Here's how the part is built. I have some questions about the finished solid (model axes, mm). A direction names the side the tool comes from. Round coordinates to 2 decimals unless told otherwise and drop trailing zeros. Order: outer loops, then holes, each group sorted by start corner. A loop starts at its lowest first (then second) coordinate and runs counter-clockwise, first axis right, second up. Notation, with made-up numbers: (20, 14.25) -> (34, 14.25) arc R9 cw to (34, 29.25) -> close; hole circle Ø2 at (-37.5, 38.25). An arc over 180 degrees is marked (long way). Use a Markdown table: item, result. Add a question column.
(1) I want a section at B-B, the plane y = 26. Please give me the cut outline in (x, z), then the cut area to 3 significant figures.
(2) On a 3-axis mill with a long thin cutter (end or side, diameter ignored), from which of +Z, -Z, +X, -X, +Y, -Y can I reach the whole of each face in a straight line? I mean faces 1 (the face through (0, 0, 0)), 2 (the face through (0, 24.1, 0)), 3 (the face through (-2.22, 29.96, 1.15)), 4 (the face through (-2.44, 13.22, -0.54)). Say none if no direction works.
(3) I want a section at D-D, the plane y = 32.1. Please give me the cut outline in (x, z), then the cut area to 3 significant figures.
(4) Thinking about a two-plate mould opening in Y: for faces 5 (the face through (-0.703, 1.663, 1.696)), 6 (the face through (0, 23.997, 3)), 7 (the face through (-1.664, 32.4, -0.954)), which applies, pulls with the +Y half, pulls with the -Y half, needs draft (parallel to the pull), parting line crosses it, or undercut?
(5) I'm going to push flat-ended pins straight in: P1, Ø1.5, axis at x = -1, y = 11, coming from the -Z side; P2, Ø3, axis at y = 12, z = 1, coming from the -X side; P3, Ø2, axis at y = 25.5, z = -3, coming from the +X side. Where does each tip first touch, or does it pass through?
(6) I want a section at C-C, the plane x = 0. Please give me the cut outline in (y, z), then the cut area to 3 significant figures.
(7) I want a section at A-A, the plane z = 0. Please give me the cut outline in (x, y).
(8) If I drill on probe 1 along Y at (x, z) = (-1.2, 0); probe 2 along X at (y, z) = (29, -0.25); probe 3 along Z at (x, y) = (2.15, 32.1), over which ranges is the centre line in solid material (lowest first)?
from build123d import *

# Parameters (mm, degrees)
SKETCH1_R           = 2.5
BOSS_EXTRUDE1_DEPTH = 36.1
SKETCH2_W           = 1.7
SKETCH2_H           = 6.818294784
CUT_EXTRUDE1_DEPTH  = 12
SKETCH3_R           = 1
CUT_EXTRUDE2_DEPTH  = 6
CHAMFER1_SIZE       = 1.1
CHAMFER1_SIZE2      = 4.2
SKETCH5_W           = 4
SKETCH5_H           = 1.5


with BuildPart() as part:
    # Sketch1 → Boss-Extrude1 (new body)
    with BuildSketch(Plane(origin=(0, 0, 0), x_dir=(1, 0, 0), z_dir=(0, 1, 0))):
        with Locations(Location((0, 0, 0), (0, 0, 270))):
            Circle(SKETCH1_R)
    extrude(amount=BOSS_EXTRUDE1_DEPTH)

    # Sketch2 → Cut-Extrude1 (cut)
    with BuildSketch(Plane(origin=(0, 36.1, 0), x_dir=(1, 0, 0), z_dir=(0, 1, 0))):
        Rectangle(SKETCH2_W, SKETCH2_H)
    extrude(amount=-CUT_EXTRUDE1_DEPTH, mode=Mode.SUBTRACT)

    # Sketch3 → Cut-Extrude2 (cut, symmetric)
    with BuildSketch(Plane(origin=(-0.85, 0, 0), x_dir=(0, 0, -1), z_dir=(1, 0, 0))):
        with Locations((0, 32.1)):
            Circle(SKETCH3_R)
    extrude(amount=CUT_EXTRUDE2_DEPTH, both=True, mode=Mode.SUBTRACT)

    # Chamfer1
    chamfer1_edges = [part.edges().sort_by_distance(p)[0] for p in [
        (0, 0, -2.5),
    ]]
    chamfer1_side = [part.faces().sort_by_distance(p)[0] for p in [
        (0, 0, 0),
    ]]
    chamfer(chamfer1_edges, length=CHAMFER1_SIZE, length2=CHAMFER1_SIZE2, reference=chamfer1_side[0])

    # Sketch5 → Revolve1 (revolve)
    with BuildSketch(Plane(origin=(0, 0, 0), x_dir=(0, 0, -1), z_dir=(1, 0, 0))):
        with Locations((-4.5, 23.247432375)):
            Rectangle(SKETCH5_W, SKETCH5_H)
    revolve(axis=Axis((0, 50, 0), (0, -1, 0)))


solid = part.part
Taken from the geometry:
| question | item | result |
|---|---|---|
| 1 | outline | (-0.85, -2.35) -> (-0.85, 2.35) arc R2.5 ccw to start; (0.85, -2.35) arc R2.5 ccw to (0.85, 2.35) -> close |
| 1 | area | 11.3 mm2 |
| 2 | face 1 | +Z, -Z, +X, -X, -Y |
| 2 | face 2 | +Z, -Z, +Y |
| 2 | face 3 | +Y |
| 2 | face 4 | -Y |
| 3 | outline | (-2.29, -1) arc R2.5 ccw to (-0.85, -2.35) -> (-0.85, -1) -> close; (-2.29, 1) -> (-0.85, 1) -> (-0.85, 2.35) arc R2.5 ccw to start; (0.85, -2.35) arc R2.5 ccw to (2.29, -1) -> (0.85, -1) -> close; (0.85, 1) -> (2.29, 1) arc R2.5 ccw to (0.85, 2.35) -> close |
| 3 | area | 4.98 mm2 |
| 4 | face 5 | pulls with the -Y half |
| 4 | face 6 | pulls with the +Y half |
| 4 | face 7 | undercut |
| 5 | P1 | stops at z = -2.49 |
| 5 | P2 | stops at x = -2.5 |
| 5 | P3 | stops at x = 1.5 |
| 6 | outline | (0, -1.4) -> (4.2, -2.5) -> (22.5, -2.5) -> (22.5, -6.5) -> (24, -6.5) -> (24, -2.5) -> (24.1, -2.5) -> (24.1, 2.5) -> (24, 2.5) -> (24, 6.5) -> (22.5, 6.5) -> (22.5, 2.5) -> (4.2, 2.5) -> (0, 1.4) -> close |
| 6 | area | 128 mm2 |
| 7 | outline | (-6.5, 22.5) -> (-2.5, 22.5) -> (-2.5, 4.2) -> (-1.4, 0) -> (1.4, 0) -> (2.5, 4.2) -> (2.5, 22.5) -> (6.5, 22.5) -> (6.5, 24) -> (2.5, 24) -> (2.5, 31.1) -> (0.85, 31.1) -> (0.85, 24.1) -> (-0.85, 24.1) -> (-0.85, 31.1) -> (-2.5, 31.1) -> (-2.5, 24) -> (-6.5, 24) -> close; (-2.5, 33.1) -> (-0.85, 33.1) -> (-0.85, 36.1) -> (-2.5, 36.1) -> close; (0.85, 33.1) -> (2.5, 33.1) -> (2.5, 36.1) -> (0.85, 36.1) -> close |
| 8 | probe 1 | y = 0 to 31.1, 33.1 to 36.1 |
| 8 | probe 2 | x = -2.49 to -0.85, 0.85 to 2.49 |
| 8 | probe 3 | z = -1.28 to -1, 1 to 1.28 |
